```python
from build123d import *

# Parameters (mm, degrees)
F0_W     = 98.2
F0_H     = 0.6
F0_W_2   = 9.6
F0_W_3   = 0.6
F0_H_2   = 40.2
F0_H_3   = 1.6
F0_H_4   = 6
F0_W_4   = 107.8
F0_W_5   = 1.6
F0_H_5   = 19.4
F0_W_6   = 67.2
F0_H_6   = 14.9
F1_DEPTH = 189.4
F2_DEPTH = 10
F3_DEPTH = 25
F4_R     = 2.5
F5_DEPTH = 7.6


with BuildPart() as f1:
    # F0 (on Front) → F1 (new body)
    with BuildSketch(Plane.XZ):
        with Locations((59.3, 49.7)):
            Rectangle(F0_W, F0_H)
        with Locations((5.4, 49.7)):
            Rectangle(F0_W_2, F0_H)
        with Locations((0.3, 29.3)):
            Rectangle(F0_W_3, F0_H_2)
        with Locations((0.3, 8.4)):
            Rectangle(F0_W_3, F0_H_3)
        with Locations((0.3, 4.6)):
            Rectangle(F0_W_3, F0_H_4)
        with Locations((0.3, 0.8)):
            Rectangle(F0_W_3, F0_H_3)
        with Locations((54.5, 0.8)):
            Rectangle(F0_W_4, F0_H_3)
        Polygon((108.4, 1.6), (108.4, 0), (110, 0), (110, 49.4), (108.4, 49.4), (108.4, 30), (108.4, 9.2), (108.4, 7.6), align=None)
        with Locations((109.2, 49.7)):
            Rectangle(F0_W_5, F0_H)
        with Locations((0.3, 49.7)):
            Rectangle(F0_W_3, F0_H)
        Polygon((0.6, 9.2), (0.6, 7.6), (108.4, 7.6), (108.4, 9.2), (78.8, 9.2), (11.6, 9.2), (10.2, 9.2), align=None)
        Polygon((0.6, 49.4), (0.6, 9.2), (10.2, 9.2), (10.2, 30), (10.2, 49.4), align=None)
        with Locations((59.3, 39.7)):
            Rectangle(F0_W, F0_H_5)
        Polygon((78.8, 9.2), (108.4, 9.2), (108.4, 30), (10.2, 30), (10.2, 9.2), (11.6, 9.2), (11.6, 24.1), (78.8, 24.1), align=None)
        with Locations((45.2, 16.65)):
            Rectangle(F0_W_6, F0_H_6)
        with Locations((54.5, 4.6)):
            Rectangle(F0_W_4, F0_H_4)
    extrude(amount=-F1_DEPTH)

    # F0 (on Front) → F2 (join)
    with BuildSketch(Plane.XZ):
        with Locations((45.2, 16.65)):
            Rectangle(F0_W_6, F0_H_6)
        Polygon((108.4, 1.6), (108.4, 0), (110, 0), (110, 49.4), (108.4, 49.4), (108.4, 30), (108.4, 9.2), (108.4, 7.6), align=None)
        with Locations((54.5, 0.8)):
            Rectangle(F0_W_4, F0_H_3)
        with Locations((109.2, 49.7)):
            Rectangle(F0_W_5, F0_H)
        with Locations((0.3, 0.8)):
            Rectangle(F0_W_3, F0_H_3)
        Polygon((0.6, 9.2), (0.6, 7.6), (108.4, 7.6), (108.4, 9.2), (78.8, 9.2), (11.6, 9.2), (10.2, 9.2), align=None)
    extrude(amount=F2_DEPTH)

    # F0 (on Front) → F3 (cut)
    with BuildSketch(Plane.XZ):
        Polygon((78.8, 9.2), (108.4, 9.2), (108.4, 30), (10.2, 30), (10.2, 9.2), (11.6, 9.2), (11.6, 24.1), (78.8, 24.1), align=None)
    extrude(amount=-F3_DEPTH, mode=Mode.SUBTRACT)

    # F4 (on face) → F5 (join, through all)
    with BuildSketch(Plane.XY.offset(9.2)):
        with Locations((6.6, -5)):
            Circle(F4_R)
    extrude(amount=-F5_DEPTH)


solid = f1.part
```
The model under review builds one solid part; all positions refer to its coordinate system, in mm. A direction names the side the tool comes from. Round coordinates to 2 decimals unless told otherwise and drop trailing zeros. Write each loop counter-clockwise with the first axis right and the second up, starting at its lowest first coordinate (ties: lowest second). Pieces come first, ordered by that corner, then holes. Notation, with made-up numbers: (-7.75, -38) - (45.25, -38) arc R11 ccw to (45.25, -32) - close; hole circle Ø1 at (76, 31.5). An arc over 180 degrees is marked (long way). Answer as CSV lines item,"result". Start each with the question number.
(1) For pin 1 Ø0.8 at (y, z) = (-7.5, 8.5) entering from -X; pin 2 Ø12 at (y, z) = (95, 21.5) entering from -X; pin 3 Ø1.5 at (x, z) = (85, 40.5) entering from -Y; pin 4 Ø5 at (x, y) = (63, -3) entering from +Z, all flat-tipped, find the tip position at first contact; note any pin that passes through.
(2) We need section B-B on y = -5. State the section outline as (x, z) points.
(3) Draft analysis for pull direction X (two halves, no side actions). For faces 1 (the flat face through (110, 91, 25)), 2 (the flat face through (55, -5, 1.6)), 3 (the flat face through (47, -10, 12)), state which applies: pulls with the +X half, pulls with the -X half, needs draft (parallel to the pull), parting line crosses it, or undercut.
(4) For faces 4 (the flat face through (54, 189.4, 25)), 5 (the flat face through (108.4, 4, 25)), 6 (the cylindrical face through (4.1, -4.9, 4.6)), list the 3-axis set-ups (+Z, -Z, +X, -X, +Y, -Y) from which the entire face can be reached by the end or side of a thin tool; tool diameter is ignored.
(5) We need section A-A on z = 4.5. State the section outline as (x, y) points.
(6) To check wall thickness, follow line 1 (Y direction, x = 65, z = 42); line 2 (Z direction, x = 11, y = 11); line 3 (Y direction, x = 105, z = 16.5). State the ranges of each line that lie inside material, in increasing order.
(7) We need section D-D on z = 38.5. State the section outline as (x, y) points.
(8) We need section C-C on x = 94. State the section outline as (y, z) points, plus the area to 3 significant figures.
Worked answers:
1,pin 1,"x = 0.6"
1,pin 2,"x = 0"
1,pin 3,"y = 0"
1,pin 4,"z = 24.1"
2,outline,"(0, 0) - (110, 0) - (110, 50) - (108.4, 50) - (108.4, 9.2) - (78.8, 9.2) - (78.8, 24.1) - (11.6, 24.1) - (11.6, 9.2) - (0.6, 9.2) - (0.6, 7.6) - (4.1, 7.6) - (4.1, 1.6) - (0, 1.6) - close; hole (9.1, 1.6) - (108.4, 1.6) - (108.4, 7.6) - (9.1, 7.6) - close"
3,face 1,"pulls with the +X half"
3,face 2,"undercut"
3,face 3,"needs draft"
4,face 4,"+Z, -Z, +X, -X, +Y"
4,face 5,"-Y"
4,face 6,"none"
5,outline,"(0, 0) - (108.4, 0) - (108.4, -10) - (110, -10) - (110, 189.4) - (0, 189.4) - close; circle Ø5 at (6.6, -5)"
6,line 1,"0 to 189.4"
6,line 2,"0 to 9.2, 30 to 50"
6,line 3,"25 to 189.4"
7,outline,"(0, 0) - (108.4, 0) - (108.4, -10) - (110, -10) - (110, 189.4) - (0, 189.4) - close"
8,outline,"(-10, 0) - (189.4, 0) - (189.4, 50) - (0, 50) - (0, 30) - (25, 30) - (25, 9.2) - (-10, 9.2) - (-10, 7.6) - (0, 7.6) - (0, 1.6) - (-10, 1.6) - close"
8,area,"8,980 mm²"
